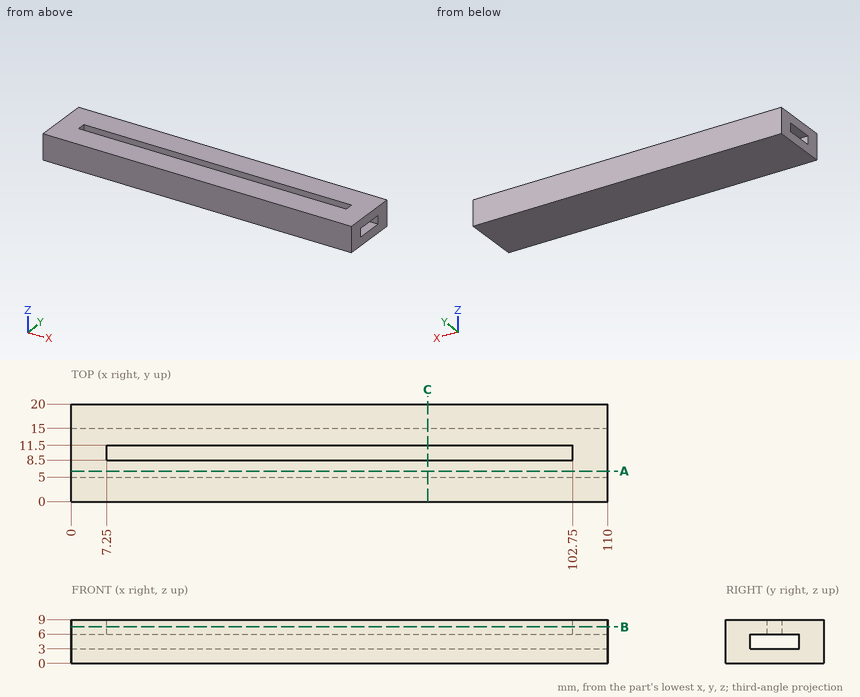
The drawing under review shows one solid part. Ordinate dimensions are in mm from its lowest x, y, z. Give positions to 0.01 mm unless a question says otherwise; leave off trailing zeros. Order: outer loops, then holes, each group sorted by start corner. A loop starts at its lowest first (then second) coordinate and runs counter-clockwise, first axis right, second up. Notation, with made-up numbers: (21.5, -6) -> (48.5, -6) arc R34 cw to (48.5, 31) -> close; hole circle Ø4 at (50.25, -6). An arc over 180 degrees is marked (long way). Write item = value, one per line. Start each with the question number.
(1) To check wall thickness, follow line 1 along Y through (x, z) = (97.5, 8); line 2 along Z through (x, y) = (18, 5.5); line 3 along Y through (x, z) = (105, 4.25). State the ranges of each line that lie inside material, in increasing order.
(2) We need section C-C on x = 73. Write out the cut boundary in (y, z), plus the area to 3 significant figures.
(3) We need section A-A on y = 6.25. Write out the cut boundary in (x, z), plus the area to 3 significant figures.
(4) We need section B-B on z = 7.5. Write out the cut boundary in (x, y).
Numbers:
q1.line_1 = 0 to 8.5, 11.5 to 20
q1.line_2 = 0 to 3, 6 to 9
q1.line_3 = 0 to 5, 15 to 20
q2.outline = (0, 0) -> (20, 0) -> (20, 9) -> (11.5, 9) -> (11.5, 6) -> (15, 6) -> (15, 3) -> (5, 3) -> (5, 6) -> (8.5, 6) -> (8.5, 9) -> (0, 9) -> close
q2.area = 141 mm^2
q3.outline = (0, 0) -> (110, 0) -> (110, 3) -> (0, 3) -> close; (0, 6) -> (110, 6) -> (110, 9) -> (0, 9) -> close
q3.area = 660 mm^2
q4.outline = (0, 0) -> (110, 0) -> (110, 20) -> (0, 20) -> close; hole (7.25, 8.5) -> (102.75, 8.5) -> (102.75, 11.5) -> (7.25, 11.5) -> close
